Build history of the part. All positions in model axes, mm. A direction names the side the tool comes from. Give positions to 0.01 mm unless a question says otherwise; leave off trailing zeros. Order: outer loops, then holes, each group sorted by start corner. A loop starts at its lowest first (then second) coordinate and runs counter-clockwise, first axis right, second up. Notation, with made-up numbers: (77.25, 86.25) -> (126.25, 86.25) arc R15 ccw to (126.25, 110.25) -> close; hole circle Ø11 at (24.25, 61). An arc over 180 degrees is marked (long way). One line per question, with ' | ' between items. Start each with the question number.
(1) Which spindle directions (+Z, -Z, +X, -X, +Y, -Y) get a long thin tool onto all of the face, cutting with end or side? Do faces 1 (the face through (2.85, 1.48, -3.01)), 2 (the face through (87.8, 2, -20)). Say none if no direction does.
(2) Drill centre lines: L1, parallel to X at y = 2.1, z = -58; L2, parallel to X at y = 1.6, z = -73; L3, parallel to Z at x = 152.5, y = 1.45. Where is each one in solid material? Low to high. Write a range as from..to.
(3) Cut at C-C (y = 0.45). Give the number of separate pieces and of enclosed holes in the cut face, then the cut area to 3 significant figures.
(4) Cut at A-A (x = 142.5). Give the cut face in (y, z).
(5) Cut at B-B (z = -63.5). Give the cut face in (x, y).
(6) Pin check, flat tips, straight feed: pin 1 Ø1.4 at (x, y) = (154.5, 2) entering from -Z; pin 2 Ø1.4 at (y, z) = (1, -6.5) entering from +X. Stop position of each tip, or through.
(7) Pull direction Z, two halves, no side cores. Call faces 3 (the face through (79, 0, -41)), 4 (the face through (86, 2, -15)), 5 (the face through (135, 2, -7)), 6 (the face through (81, 1, -80)): +Z half, -Z half, draft (parallel to the pull), parting line (faces both ways), or undercut.
from build123d import *

# Parameters (mm, degrees)
BOSS_EXTRU_1_DEPTH      = 3
ESQUISSE4_W             = 10
ESQUISSE4_H             = 2.8
ENL_V_MAT_EXTRU_2_DEPTH = 179.910592196
ESQUISSE5_W             = 2.8
ESQUISSE5_H             = 10
ENL_V_MAT_EXTRU_3_DEPTH = 179.910592196


with BuildPart() as part:
    # Esquisse2 → Boss.-Extru.1 (new body)
    with BuildSketch(Plane(origin=(0, 0, 0), x_dir=(1, 0, 0), z_dir=(0, 1, 0))):
        with BuildLine():
            Line((10, 0), (150, 0))
            ThreePointArc((150, 0), (157.071067812, 2.928932188), (160, 10))
            Line((160, 10), (160, 70))
            ThreePointArc((160, 70), (157.071067812, 77.071067812), (150, 80))
            Line((150, 80), (10, 80))
            ThreePointArc((10, 80), (2.928932188, 77.071067812), (0, 70))
            Line((0, 70), (0, 10))
            ThreePointArc((0, 10), (2.928932188, 2.928932188), (10, 0))
        make_face()
    extrude(amount=BOSS_EXTRU_1_DEPTH)

    # Esquisse4 → Enlèv. mat.-Extru.2 (cut, through all)
    with BuildSketch(Plane(origin=(0, 3, 0), x_dir=(1, 0, 0), z_dir=(0, 1, 0))):
        with Locations((140, 73.6)):
            Rectangle(ESQUISSE4_W, ESQUISSE4_H)
        with Locations((100, 73.6)):
            Rectangle(ESQUISSE4_W, ESQUISSE4_H)
        with Locations((100, 6.6)):
            Rectangle(ESQUISSE4_W, ESQUISSE4_H)
        with Locations((140, 6.6)):
            Rectangle(ESQUISSE4_W, ESQUISSE4_H)
    extrude(amount=-ENL_V_MAT_EXTRU_2_DEPTH, mode=Mode.SUBTRACT)

    # Esquisse5 → Enlèv. mat.-Extru.3 (cut, through all)
    with BuildSketch(Plane(origin=(0, 3, 0), x_dir=(1, 0, 0), z_dir=(0, 1, 0))):
        with Locations((153.6, 60)):
            Rectangle(ESQUISSE5_W, ESQUISSE5_H)
        with Locations((86.4, 60)):
            Rectangle(ESQUISSE5_W, ESQUISSE5_H)
        with Locations((86.4, 20)):
            Rectangle(ESQUISSE5_W, ESQUISSE5_H)
        with Locations((153.6, 20)):
            Rectangle(ESQUISSE5_W, ESQUISSE5_H)
    extrude(amount=-ENL_V_MAT_EXTRU_3_DEPTH, mode=Mode.SUBTRACT)


solid = part.part
Result set:
1) face 1: +Z, -X, +Y, -Y | face 2: +Y, -Y
2) L1: x = 0..85, 87.8..152.2, 155..160 | L2: x = 0.46..95, 105..135, 145..159.54 | L3: z = -79.68..-65, -55..-25, -15..-0.32
3) separate pieces: 1 | enclosed holes: 8 | area: 12,500 mm2
4) outline: (0, -80) -> (3, -80) -> (3, -75) -> (0, -75) -> close; (0, -72.2) -> (3, -72.2) -> (3, -8) -> (0, -8) -> close; (0, -5.2) -> (3, -5.2) -> (3, 0) -> (0, 0) -> close
5) outline: (0, 0) -> (85, 0) -> (85, 3) -> (0, 3) -> close; (87.8, 0) -> (152.2, 0) -> (152.2, 3) -> (87.8, 3) -> close; (155, 0) -> (160, 0) -> (160, 3) -> (155, 3) -> close
6) pin 1: stops at z = -79.25 | pin 2: stops at x = 159.6
7) face 3: draft | face 4: undercut | face 5: undercut | face 6: -Z half
